Autodesk Inventor part; units mm, degrees
ref_plane "YZ Plane" through (0, 0, 0) normal (1, 0, 0) x (0, 1, 0)
ref_plane "XZ Plane" through (0, 0, 0) normal (0, 1, 0) x (-1, 0, 0)
ref_plane "XY Plane" through (0, 0, 0) normal (0, 0, 1) x (1, 0, 0)
sketch "Boceto1" plane through (0, 0, 0) normal (0, 1, 0) x (-1, 0, 0)
  line L0 (20.25, -43.5) -> (-20.25, -43.5)
  line L1 (-20.25, -43.5) -> (-20.25, 43.5)
  line L2 (-20.25, 43.5) -> (20.25, 43.5)
  line L3 (20.25, 43.5) -> (20.25, -43.5)
  line L4 (20.25, -43.5) -> (-20.25, 43.5) construction
  line L5 (-20.25, -43.5) -> (20.25, 43.5) construction
  line L6 (25.25, -48.5) -> (-25.25, -48.5)
  line L7 (-25.25, -48.5) -> (-25.25, 48.5)
  line L8 (-25.25, 48.5) -> (25.25, 48.5)
  line L9 (25.25, 48.5) -> (25.25, -48.5)
  line L10 (20.25, 43.5) -> (-20.25, 43.5)
  line L11 (-20.25, 43.5) -> (-20.25, 14)
  line L12 (-20.25, 14) -> (20.25, 14)
  line L13 (20.25, 14) -> (20.25, 43.5)
  line L14 (25.25, 14) -> (-25.25, 14)
  line L15 (21.25, -44.5) -> (-21.25, -44.5)
  line L16 (-21.25, -44.5) -> (-21.25, 44.5)
  line L17 (-21.25, 44.5) -> (21.25, 44.5)
  line L18 (21.25, 44.5) -> (21.25, -44.5)
  line L19 (8.5, 14) -> (-8.5, 14)
  line L20 (-8.5, 14) -> (-8.5, 16)
  line L21 (-8.5, 16) -> (8.5, 16)
  line L22 (8.5, 16) -> (8.5, 14)
  point P0 (0, 0)
  point P1 (0, 0)
  point P2 (-20.25, 14)
  point P3 (-20.25, 14)
  point P4 (20.25, 14)
  point P5 (20.25, 14)
  point P6 (0, 14)
  dimension "d0" = 40.5
  dimension "d1" = 87
  dimension "d2" = 5
  dimension "d3" = 29.5
  dimension "d19" = 1
  dimension "d29" = 17
  dimension "d32" = 2
extrude "Extrusión4" add sketch "Boceto1" against normal blind 7.5 contours L3 L14 L18 L15 L16 L1 L0 | L3 L2 L1 L14 L16 L17 L18 | L18 L17 L16 L14 L7 L8 L9 | L14 L9 L6 L7 L16 L15 L18
extrude "Extrusión5" add sketch "Boceto1" along normal blind 1 contours L3 L14 L18 L15 L16 L1 L0 | L12 L22 L21 L20 L1 L2 L3 | L3 L2 L1 L14 L16 L17 L18 | L12 L20 L21 L22 | L18 L17 L16 L14 L7 L8 L9 | L14 L9 L6 L7 L16 L15 L18
fillet "Empalme2" radius 4 4 edges at (-20.25, -3.25, -43.5) (20.25, -3.25, -43.5) (20.25, -3.75, 43.5) (-20.25, -3.75, 43.5)
fillet "Empalme3" radius 2 1 edges at (0, 0, 14)
sketch "Boceto2" plane through (0, 0, 0) normal (1, 0, 0) x (0, 1, 0)
  line L0 (1, 14) -> (1, -39.5) construction
  line L1 (1, 14) -> (4, 14)
  line L2 (4, 14) -> (4, 9)
  line L3 (1, -3.5) -> (11, -3.5) construction
  line L4 (4, 14) -> (11, -3.5)
  line L5 (11, -3.5) -> (9.143, 1.1424)
  line L6 (0, 15) -> (0, -39.5) construction
  line L7 (1, -43.5) -> (1, -39.5) construction
  line L8 (1, -43.5) -> (13, -43.5)
  line L9 (13, -43.5) -> (10.5, -43.5)
  line L10 (1, -43.5) -> (13, -43.5)
  line L11 (13, -43.5) -> (13, -44.5)
  line L12 (13, -44.5) -> (1, -44.5)
  line L13 (1, -44.5) -> (1, -43.5)
  line L14 (10.5, -43.5) -> (10.5, -38.5)
  line L15 (10.5, -38.5) -> (9.5, -38.5)
  line L16 (9.5, -38.5) -> (9.5, -43.5)
  line L17 (9.5, -43.5) -> (10.5, -43.5)
  line L18 (10.5, -43.5) -> (10.5, -38.5)
  line L19 (13, -43.5) -> (13, -3.5) construction
  line L20 (13, -43.5) -> (13, -36.5) construction
  line L21 (13, -36.5) -> (12, -36.5) construction
  line L22 (13, -36.5) -> (13, -43.5)
  line L23 (11, -3.5) -> (13, -36.5)
  line L24 (1, 14) -> (-1, 14)
  line L25 (-1, 14) -> (-1, 43.5)
  line L26 (0, 43.5) -> (-7.5, 43.5)
  line L27 (0, 39.5) -> (0, 15.7321)
  line L28 (-7.5, 48.5) -> (-7.5, -48.5) construction
  line L29 (1, -43.5) -> (-7.5, -43.5)
  line L30 (-7.5, -43.5) -> (-7.5, -44.5)
  line L31 (-7.5, -44.5) -> (1, -44.5)
  line L32 (1, -44.5) -> (1, -43.5)
  point P0 (0, 0)
  dimension "d22" = 3
  dimension "d23" = 5
  dimension "d24" = 10
  dimension "d25" = 17.5
  dimension "d26" = 5
  dimension "d33" = 12
  dimension "d36" = 1
  dimension "d37" = 5
  dimension "d38" = 1
  dimension "d39" = 40
  dimension "d40" = 7
  dimension "d41" = 1
  dimension "d48" = 1
feature "Barrido1" [suppressed]
extrude "Extrusión7" [suppressed]
extrude "Extrusión8" cut sketch "Boceto1" along normal blind 10 contours L12 L20 L21 L22
extrude "Extrusión9" cut sketch "Boceto2" along normal mid plane 17 contours L13 L31 L30 L29
properties part number "manija_puerta_marco_front_right_v3"
Can you work these out from the model? Positions are in its coordinate system, mm. A direction names the side the tool comes from. Coordinates: 2 decimals unless noted, no trailing zeros. Write each loop counter-clockwise with the first axis right and the second up, starting at its lowest first coordinate (ties: lowest second). Pieces come first, ordered by that corner, then holes. Notation, with made-up numbers: (51, 53.5) -> (68, 53.5) arc R14 cw to (68, 60.5) -> close; hole circle Ø9 at (12.25, 35.25). An arc over 180 degrees is marked (long way). Write each question's results on one line, items separated by ' | '. Start each with the question number.
Q1. Imagine slicing it at A-A (x = 10.5). Write out the boundary of the cut face in (y, z).
Q2. If I drill on probe 1 along X at (y, z) = (-4.5, -34.5); probe 2 along Z at (x, y) = (0.5, -6); probe 3 along X at (y, z) = (-6.75, -44), over which ranges is the centre line in solid material (lowest first)?
Q3. We'd pull the mould along Z, two halves only. Please class faces 1 (the face through (14.457, 0.261, 14.745)), 2 (the face through (0, -3, 48.5)), 3 (the face through (-25.25, -3, 1)): +Z half, -Z half, draft (parallel to the pull), parting line (faces both ways), or undercut.
Q4. Imagine slicing it at C-C (y = -3.5). Write out the boundary of the cut face in (x, z), then the cut area to 3 significant figures.
Q5. On a 3-axis mill with a long thin cutter (end or side, diameter ignored), from which of +Z, -Z, +X, -X, +Y, -Y can I reach the whole of each face in a straight line? I mean faces 4 (the face through (12, -3, -43.5)), 5 (the face through (25.25, -3, -1)), 6 (the face through (0, -4, 43.5)). Say none if no direction works.
Q6. Imagine slicing it at D-D (x = -4). Write out the boundary of the cut face in (y, z).
Q7. I'm going to push a flat-ended pin straight in: pin 1 (14 mm diameter, centred on x = 4.5, z = 27, fed in from -Y). Where does the tip first touch, or does it pass through?
Q8. Imagine slicing it at B-B (z = -36.5). Write out the boundary of the cut face in (x, y).
Taken from the geometry:
1) outline: (-7.5, -48.5) -> (1, -48.5) -> (1, -43.5) -> (-7.5, -43.5) -> close; (-7.5, 43.5) -> (0, 43.5) -> (0, 15.73) arc R2 ccw to (1, 14) -> (1, 48.5) -> (-7.5, 48.5) -> close
2) probe 1: x = -25.25 to -20.25, 20.25 to 25.25 | probe 2: z = -48.5 to -44.5, 43.5 to 48.5 | probe 3: x = -25.25 to -8.5, 8.5 to 25.25
3) face 1: undercut | face 2: +Z half | face 3: draft
4) outline: (-25.25, -48.5) -> (25.25, -48.5) -> (25.25, 48.5) -> (-25.25, 48.5) -> close; hole (-20.25, -39.5) arc R4 ccw to (-16.25, -43.5) -> (-8.5, -43.5) -> (-8.5, -44.5) -> (8.5, -44.5) -> (8.5, -43.5) -> (16.25, -43.5) arc R4 ccw to (20.25, -39.5) -> (20.25, 39.5) arc R4 ccw to (16.25, 43.5) -> (-16.25, 43.5) arc R4 ccw to (-20.25, 39.5) -> close | area: 1,370 mm^2
5) face 4: +Y, -Y | face 5: +Z, -Z, +X, +Y, -Y | face 6: -Y
6) outline: (-7.5, -48.5) -> (1, -48.5) -> (1, -44.5) -> (-7.5, -44.5) -> close; (-7.5, 43.5) -> (0, 43.5) -> (0, 16) -> (1, 16) -> (1, 48.5) -> (-7.5, 48.5) -> close
7) pin 1: stops at y = 0
8) outline: (-25.25, -7.5) -> (-20.25, -7.5) -> (-20.25, 1) -> (-25.25, 1) -> close; (20.25, -7.5) -> (25.25, -7.5) -> (25.25, 1) -> (20.25, 1) -> close
